```python
from build123d import *

# Parameters (mm, degrees)
SKETCH1_R           = 5.8
BOSS_EXTRUDE1_DEPTH = 49
SHELL2_T            = -1
SKETCH5_R           = 2
CUT_EXTRUDE1_DEPTH  = 50.681787407
CIRPATTERN1_COUNT   = 2
CIRPATTERN1_ANGLE   = 90
CUT_EXTRUDE2_REACH  = 51.682
SKETCH6_R           = 1.5


with BuildPart() as part:
    # Sketch1 → Boss-Extrude1 (new body)
    with BuildSketch(Plane(origin=(0, 0, 0), x_dir=(1, 0, 0), z_dir=(0, 1, 0))):
        with Locations(Location((0, 0, 0), (0, 0, 270))):
            Circle(SKETCH1_R)
    extrude(amount=BOSS_EXTRUDE1_DEPTH)

    # Shell2
    shell2_openings = [part.faces().sort_by_distance(p)[0] for p in [
        (0, 0, 0),
    ]]
    offset(amount=SHELL2_T, openings=shell2_openings, kind=Kind.INTERSECTION)

    # Sketch5 → Cut-Extrude1 (cut, symmetric)
    with BuildSketch(Plane.XY):
        with Locations((0, 40)):
            Circle(SKETCH5_R)
    cut_extrude1 = extrude(amount=CUT_EXTRUDE1_DEPTH, both=True, mode=Mode.SUBTRACT)

    # CirPattern1: Cut-Extrude1 ×2 about axis
    cirpattern1_axis = Axis((0, 49, 0), (0, -1, 0))
    for i in range(1, CIRPATTERN1_COUNT):
        add(cut_extrude1.rotate(cirpattern1_axis, i * CIRPATTERN1_ANGLE / (CIRPATTERN1_COUNT - 1)), mode=Mode.SUBTRACT)

    # Sketch6 → Cut-Extrude2 (cut, up to next)
    with BuildSketch(Plane(origin=(0, 49, 0), x_dir=(1, 0, 0), z_dir=(0, 1, 0)), mode=Mode.PRIVATE) as cut_extrude2_sk1:
        with Locations(Location((0, 0, 0), (0, 0, 270))):
            Circle(SKETCH6_R)
    cut_extrude2_tool1 = extrude(cut_extrude2_sk1.sketch, amount=-CUT_EXTRUDE2_REACH, mode=Mode.PRIVATE) & part.part
    add(cut_extrude2_tool1.solids().sort_by_distance((0, 49, 0))[0], mode=Mode.SUBTRACT)


solid = part.part
```
Verification items for the finished model (mm, model axes). A direction names the side the tool comes from. Round coordinates to 2 decimals unless told otherwise and drop trailing zeros. Loops run counter-clockwise (first coordinate to the right, second up) from the corner with the lowest first, then second, coordinate; pieces in that order, holes last. Notation, with made-up numbers: (29.25, 17) -> (72.25, 17) arc R20 cw to (72.25, 53) -> close; hole circle Ø7 at (-30.5, 47.5). An arc over 180 degrees is marked (long way). Answer as a JSON object with one key per item and string values.
Q1. Access from +Z, -Z, +X, -X, +Y, -Y to the whole of each face (thin tool, end or side, straight path). Record for faces 5 (the cylindrical face through (-5.146, 24.157, 2.676)), 6 (the flat face through (0, 48, 2)).
Data:
{"face 5": "+Y, -Y", "face 6": "-Y"}
Q2. Section check C-C (y = 20). Record the boundary of the cut face in (x, z), then the cut area to 3 significant figures.
Data:
{"outline": "circle Ø11.6 at (0, 0); hole circle Ø9.6 at (0, 0)", "area": "33.3 mm2"}
Q3. Section check B-B (x = 0). Record the boundary of the cut face in (y, z), then the cut area to 3 significant figures.
Data:
{"outline": "(0, -5.8) -> (38, -5.8) -> (38, -4.8) -> (0, -4.8) -> close; (0, 4.8) -> (38, 4.8) -> (38, 5.8) -> (0, 5.8) -> close; (42, -5.8) -> (49, -5.8) -> (49, -1.5) -> (48, -1.5) -> (48, -4.8) -> (42, -4.8) -> close; (42, 4.8) -> (48, 4.8) -> (48, 1.5) -> (49, 1.5) -> (49, 5.8) -> (42, 5.8) -> close", "area": "96.6 mm2"}
Q4. Go/stop test with flat-tipped pins: P1, Ø4, axis at x = -1, y = 40.5, coming from the -Z side; P2, Ø3.5, axis at x = 0, z = 0, coming from the -Y side; P3, Ø6, axis at x = -4.5, y = 9, coming from the +Z side. Record where each tip stops, or that it passes through.
Data:
{"P1": "stops at z = -5.8", "P2": "stops at y = 48", "P3": "stops at z = 5.6"}
Q5. Scan lines: line 1 (X direction, y = 48.4, z = 0); line 2 (Y direction, x = 0, z = 5.35); line 3 (Y direction, x = -1.25, z = 2.5). Record each from-to range of solid material in increasing order. Write a range as from..to.
Data:
{"line 1": "x = -5.8..-1.5, 1.5..5.8", "line 2": "y = 0..38, 42..49", "line 3": "y = 48..49"}
Q6. Section check D-D (y = 40). Record the boundary of the cut face in (x, z).
Data:
{"outline": "(-5.44, -2) arc R5.8 ccw to (-2, -5.44) -> (-2, -4.36) arc R4.8 cw to (-4.36, -2) -> close; (-5.44, 2) -> (-4.36, 2) arc R4.8 cw to (-2, 4.36) -> (-2, 5.44) arc R5.8 ccw to start; (2, -5.44) arc R5.8 ccw to (5.44, -2) -> (4.36, -2) arc R4.8 cw to (2, -4.36) -> close; (2, 4.36) arc R4.8 cw to (4.36, 2) -> (5.44, 2) arc R5.8 ccw to (2, 5.44) -> close"}
Q7. Section check A-A (z = 0). Record the boundary of the cut face in (x, y), then the cut area to 3 significant figures.
Data:
{"outline": "(-5.8, 0) -> (-4.8, 0) -> (-4.8, 38) -> (-5.8, 38) -> close; (-5.8, 42) -> (-4.8, 42) -> (-4.8, 48) -> (-1.5, 48) -> (-1.5, 49) -> (-5.8, 49) -> close; (1.5, 48) -> (4.8, 48) -> (4.8, 42) -> (5.8, 42) -> (5.8, 49) -> (1.5, 49) -> close; (4.8, 0) -> (5.8, 0) -> (5.8, 38) -> (4.8, 38) -> close", "area": "96.6 mm2"}
Q8. Draft check along Y on faces 1 (the cylindrical face through (5, 38, 0)), 2 (the flat face through (5, 0, 1)), 3 (the cylindrical face through (0.211, 23.664, -4.795)), 4 (the cylindrical face through (-5, 40, -2)). Enter one of: pulls with the +Y half, pulls with the -Y half, needs draft (parallel to the pull), parting line crosses it, or undercut.
Data:
{"face 1": "undercut", "face 2": "pulls with the -Y half", "face 3": "needs draft", "face 4": "undercut"}
